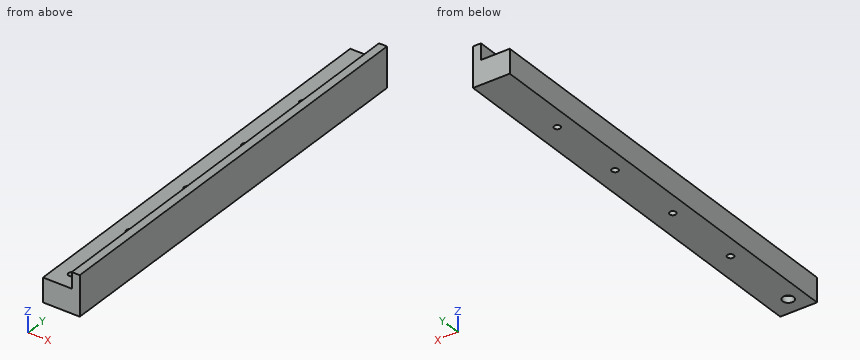
Autodesk Fusion 360 part; units mm, degrees
sketch "Szkic1" plane through (0, 0, 0) normal (0, 0, 1) x (1, 0, 0)
  line L0 (45, 135) -> (-35, 135)
  line L1 (-35, 135) -> (-35, -130)
  line L2 (-35, -130) -> (45, -130)
  circle A0 centre (25, -120) radius 1.75
  circle A1 centre (-25, -120) radius 1.75
  circle A2 centre (-25, -70) radius 1.75
  circle A3 centre (-25, -20) radius 1.75
  circle A4 centre (-25, 30) radius 1.75
  circle A5 centre (-25, 80) radius 1.75
  circle A6 centre (-15, 125) radius 3.5
  circle A7 centre (20, 125) radius 3.5
  circle A8 centre (20, 105) radius 3.5
  circle A9 centre (-15, 105) radius 3.5
  line L3 (45, -130) -> (45, -105)
  line L4 (45, -105) -> (-35, -105)
  line L5 (-35, -105) -> (-35, -130)
  line L6 (-35, -130) -> (45, -130)
  line L7 (-35, -130) -> (-17, -130)
  line L8 (-17, -130) -> (-17, 135)
  line L9 (-17, 135) -> (-35, 135)
  line L10 (-35, 135) -> (-35, -130)
  line L11 (-17, 135) -> (-17, -130)
  line L12 (-17, -130) -> (-12, -130)
  line L13 (-12, -130) -> (-12, 135)
  line L14 (-12, 135) -> (-17, 135)
  dimension "d1" = 5
extrude "Wyciągnięcie proste1" add sketch "Szkic1" along normal blind 25 contours L0 A6 L8 L11 L13 L14 | A6 L8 L11 L13 | A6 A9 L8 L11 L13 | A9 L8 L11 L13 | A9 L4 L8 L11 L13
extrude "Wyciągnięcie proste2" add sketch "Szkic1" along normal blind 15 contours L0 L1 A6 A9 L4 L8 L9 L10 L11 | A6 L8 L11 | A9 L8 L11
extrude "Wyciągnięcie proste3" add 1 faces at (-21.3333, -105, 5) along direction (0, -1, 0) blind 26
extrude "Wyciągnięcie proste4" cut sketch "Szkic1" along normal blind 37 contours A1
sketch "Szkic2" plane through (0, 0, 0) normal (0, 0, -1) x (1, 0, 0)
  circle A0 centre (-25, 120) radius 1.75
  circle A1 centre (-25, -30) radius 1.75
  circle A2 centre (-25, -80) radius 1.75
  circle A3 centre (-25, 20) radius 1.75
  circle A4 centre (-25, 70) radius 1.75
  line L0 (-12, -135) -> (-12, 131)
  line L1 (-12, 131) -> (-35, 131)
  line L2 (-35, 131) -> (-35, -135)
  line L3 (-35, -135) -> (-12, -135)
  circle A5 centre (-25, 120) radius 2
  circle A6 centre (-25, 120) radius 3.5
  circle A7 centre (-25, 70) radius 2
  circle A8 centre (-25, 20) radius 2
  circle A9 centre (-25, -30) radius 2
  circle A10 centre (-25, -80) radius 2
  dimension "d10" = 4
  dimension "d11" = 7
  dimension "d12" = 4
  dimension "d13" = 4
  dimension "d14" = 4
  dimension "d15" = 4
extrude "Wyciągnięcie proste5" cut sketch "Szkic2" against normal blind 100 contours A5 | A7 | A8 | A9 | A10
extrude "Wyciągnięcie proste6" cut sketch "Szkic2" against normal blind 4 contours A6
Source: CAD feature listing. Evaluate the final solid. Frame: model axes, mm. Round coordinates to 2 decimals unless told otherwise and drop trailing zeros. Write each loop counter-clockwise with the first axis right and the second up, starting at its lowest first coordinate (ties: lowest second). Pieces come first, ordered by that corner, then holes. Notation, with made-up numbers: (-6, -18) - (17, -18) arc R18 cw to (17, -7) - close; hole circle Ø3 at (66, 45). An arc over 180 degrees is marked (long way). Use CSV: the item, a comma, the result in double quotes. Start each with the question number.
(1) Cut plane A-A, the plane z = 18.5. Return loops of the section in (x, y).
(2) Material intervals for probe 1 along Y at (x, z) = (-25, 5); probe 2 along X at (y, z) = (-70, 5.5); probe 3 along X at (y, z) = (70, 15.25), sorted ascending. Write a range as [from, to].
(3) First-contact query: pin 1 Ø3.5 at (x, y) = (-26, -120) entering from -Z. Flat tip, straight axial feed; report the tip coordinate or a pass-through.
(4) Cut plane B-B, the plane y = -7.5. Return loops of the section in (x, z), and give its area (3 significant figures).
Geometry says:
1,outline,"(-17, -131) - (-12, -131) - (-12, 135) - (-17, 135) - close"
2,probe 1,"[-131, -122], [-118, -72], [-68, -22], [-18, 28], [32, 78], [82, 135]"
2,probe 2,"[-35, -27], [-23, -12]"
2,probe 3,"[-17, -12]"
3,pin 1,"z = 4"
4,outline,"(-35, 0) - (-12, 0) - (-12, 25) - (-17, 25) - (-17, 15) - (-35, 15) - close"
4,area,"395 mm²"
